Read the model definition and answer for the solid it produces. Units are mm, in the model's axes. Face numbers are marked on the shaded views. A direction names the side the tool comes from. Coordinates: 2 decimals unless noted, no trailing zeros. Write each loop counter-clockwise with the first axis right and the second up, starting at its lowest first coordinate (ties: lowest second). Pieces come first, ordered by that corner, then holes. Notation, with made-up numbers: (56, 60.5) -> (78, 60.5) arc R36 cw to (78, 98.5) -> close; hole circle Ø10 at (-30, 53.5). An arc over 180 degrees is marked (long way). Use CSV: the item, a comma, the result in double quotes. Start each with the question number.
from build123d import *

# Parameters (mm, degrees)
AUFSATZ_LINEAR_AUSTRAGEN1_DEPTH = 3
AUFSATZ_LINEAR_AUSTRAGEN2_DEPTH = 8
SCHNITT_LINEAR_AUSTRAGEN1_DEPTH = 19
F_4_0_4_DURCHMESSER_BOHRUNG1_D  = 4
SKIZZE7_W                       = 12
SKIZZE7_H                       = 3
SCHNITT_LINEAR_AUSTRAGEN2_DEPTH = 4


with BuildPart() as part:
    # Skizze1 → Aufsatz-Linear austragen1 (new body)
    with BuildSketch(Plane(origin=(0, 0, 0), x_dir=(1, 0, 0), z_dir=(0, 1, 0))):
        Polygon((9, -13.5), (-9, -13.5), (-9, 2.5), (-7, 13.5), (7, 13.5), (9, 2.5), align=None)
    extrude(amount=AUFSATZ_LINEAR_AUSTRAGEN1_DEPTH)

    # Skizze2 → Aufsatz-Linear austragen2 (add)
    with BuildSketch(Plane(origin=(0, 3, 0), x_dir=(1, 0, 0), z_dir=(0, 1, 0))):
        Polygon((-9, 2.5), (-7, 13.5), (7, 13.5), (9, 2.5), (5.454545455, 2.5), (4, 10.5), (-4, 10.5), (-5.454545455, 2.5), align=None)
    extrude(amount=AUFSATZ_LINEAR_AUSTRAGEN2_DEPTH)

    # Skizze3 → Schnitt-Linear austragen1 (cut, through all)
    with BuildSketch(Plane.ZY.offset(9)):
        Polygon((-2.5, 3), (-10.5, 11), (-10.5, 11.548475308), (-1.609095569, 11.548475308), (-1.609095569, 3.67540056), align=None)
    extrude(amount=-SCHNITT_LINEAR_AUSTRAGEN1_DEPTH, mode=Mode.SUBTRACT)

    # Ø4.0 (4) Durchmesser Bohrung1 (through all)
    with Locations(Plane(origin=(0, 0, -13.5), x_dir=(-1, 0, 0), z_dir=(0, 0, -1))):
        with Locations((0, 7)):
            Hole(F_4_0_4_DURCHMESSER_BOHRUNG1_D / 2)

    # Skizze7 → Schnitt-Linear austragen2 (cut, through all)
    with BuildSketch(Plane(origin=(0, 3, 0), x_dir=(1, 0, 0), z_dir=(0, 1, 0))):
        with Locations((0, -9)):
            Rectangle(SKIZZE7_W, SKIZZE7_H)
        with Locations((0, -1)):
            Rectangle(SKIZZE7_W, SKIZZE7_H)
    extrude(amount=-SCHNITT_LINEAR_AUSTRAGEN2_DEPTH, mode=Mode.SUBTRACT)


solid = part.part
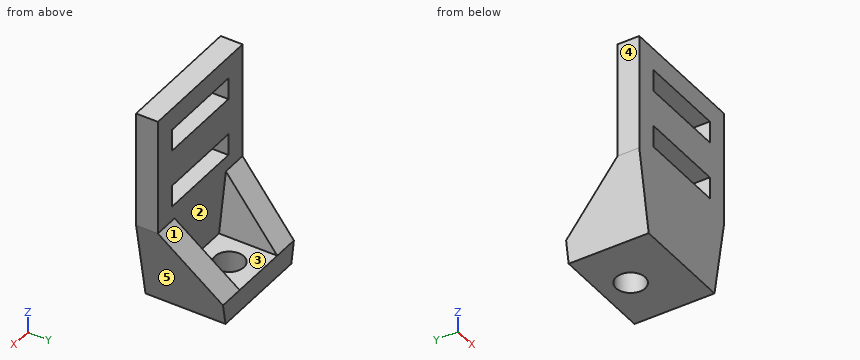
1) Find the intervals of material crossed by line 1 along Y through (x, z) = (0, -12.55); line 2 along Z through (x, y) = (3, 1); line 3 along Y through (x, z) = (2.25, 4.25), in increasing order.
2) The mould has two halves that part along X. Classify the marked faces 3, 4 and 5: pulls with the +X half, pulls with the -X half, needs draft (parallel to the pull), parting line crosses it, or undercut.
3) Which of the six approach directions +Z, -Z, +X, -X, +Y, -Y give full straight-line access (tool end or side, diameter ignored) to the marked faces 1 and 2?
4) Section C-C, the plane y = 5.5 is taken. Give the vertices of the cut face in (x, z).
5) Section D-D, the plane z = -11.5 is taken. Give the vertices of the cut face in (x, y), plus the area to 3 significant figures.
6) Section A-A, the plane x = 2.5 is taken. Give the vertices of the cut face in (y, z).
7) Section B-B, the plane x = -1 is taken. Give the vertices of the cut face in (y, z).
8) Each of these flat-tipped pins is pushed along its axis until it touches: pin 1 (1.5 mm diameter, centred on x = 0, z = -1, fed in from +Y); pin 2 (5 mm diameter, centred on y = 8.5, z = -9, fed in from -X). Where does it stop, or does it pass through?
The answers:
1,line 1,"y = 0 to 5, 9 to 11"
1,line 2,"z = -13.5 to -0.5, 2.5 to 7.5, 10.5 to 13.5"
1,line 3,"y = 0 to 3"
2,face 3,"undercut"
2,face 4,"pulls with the -X half"
2,face 5,"pulls with the +X half"
3,face 1,"+Z, +X, -X, +Y"
3,face 2,"+Z, +Y"
4,outline,"(-8.55, -5) -> (-7, -13.5) -> (-1.32, -13.5) -> (-1.32, -10.5) -> (-4, -10.5) -> (-5, -5) -> close; (1.32, -13.5) -> (7, -13.5) -> (8.55, -5) -> (5, -5) -> (4, -10.5) -> (1.32, -10.5) -> close"
5,outline,"(-7.36, 0) -> (7.36, 0) -> (7.36, 11) -> (-7.36, 11) -> close; hole circle Ø4 at (0, 7)"
5,area,"149 mm^2"
6,outline,"(0, -13.5) -> (11, -13.5) -> (11, -10.5) -> (3, -10.5) -> (3, -0.5) -> (0, -0.5) -> close; (0, 2.5) -> (3, 2.5) -> (3, 7.5) -> (0, 7.5) -> close; (0, 10.5) -> (3, 10.5) -> (3, 13.5) -> (0, 13.5) -> close"
7,outline,"(0, -13.5) -> (5.27, -13.5) -> (5.27, -10.5) -> (3, -10.5) -> (3, -0.5) -> (0, -0.5) -> close; (0, 2.5) -> (3, 2.5) -> (3, 7.5) -> (0, 7.5) -> close; (0, 10.5) -> (3, 10.5) -> (3, 13.5) -> (0, 13.5) -> close; (8.73, -13.5) -> (11, -13.5) -> (11, -10.5) -> (8.73, -10.5) -> close"
8,pin 1,"stops at y = 3"
8,pin 2,"stops at x = -8.22"
